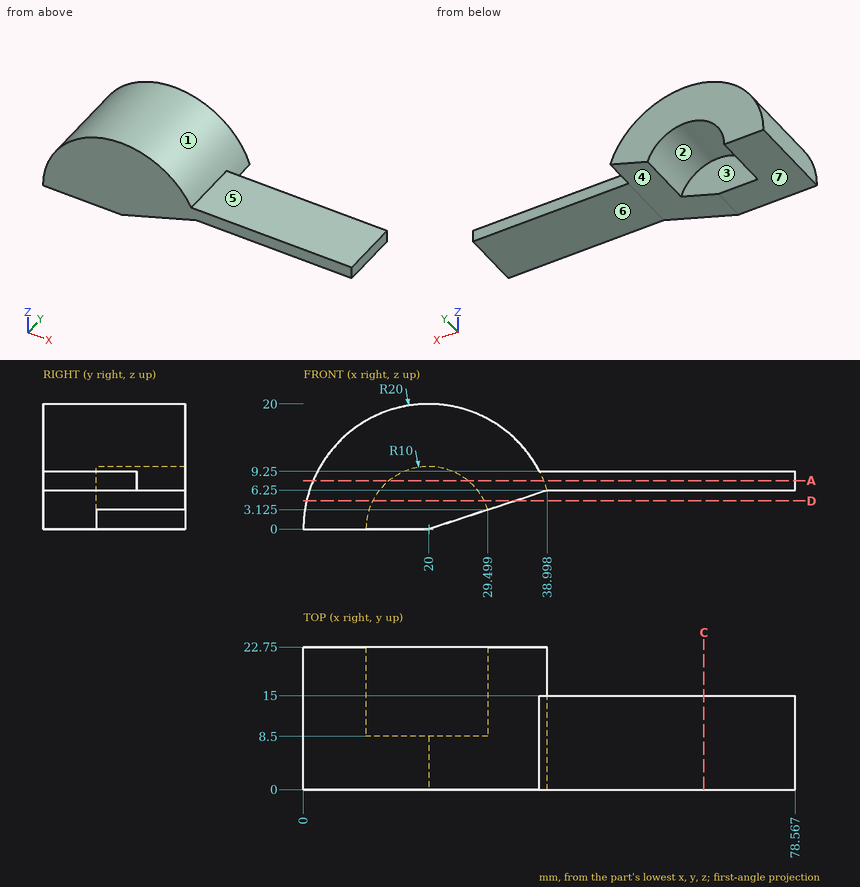
Verification items for this drawing (mm, ordinates from the low corner). A direction names the side the tool comes from. Round coordinates to 2 decimals unless told otherwise and drop trailing zeros. Write each loop counter-clockwise with the first axis right and the second up, starting at its lowest first coordinate (ties: lowest second). Pieces come first, ordered by that corner, then holes. Notation, with made-up numbers: (-2, -0.75) - (16, -0.75) arc R14 ccw to (16, 18.25) - close; hole circle Ø6 at (-25.5, 37). An arc over 180 degrees is marked (long way). One line per item, written item: value.
1. Depth check by flat-ended pin: pin 1 Ø4.5 at (x, y) = (66, 8) entering from -Z; pin 2 Ø1.5 at (x, y) = (30, 2.5) entering from +Z; pin 3 Ø8 at (x, z) = (43, 7) entering from +Y; pin 4 Ø8 at (x, z) = (16, 6.5) entering from +Y. Enter the tip coordinate at first touch or a pass-through.
The answers:
pin 1: stops at z = 6.25
pin 2: stops at z = 17.73
pin 3: stops at y = 15
pin 4: stops at y = 22.75
2. Cross-section at A-A on z = 7.75. Record the boundary of the cut face in (x, y).
The answers:
outline: (1.56, 0) - (78.57, 0) - (78.57, 15) - (38.44, 15) - (38.44, 22.75) - (26.32, 22.75) - (26.32, 8.5) - (13.68, 8.5) - (13.68, 22.75) - (1.56, 22.75) - close
3. Set-up check for the marked faces 5, 6 and 7: record each of +Z, -Z, +X, -X, +Y, -Y from which the full face is reachable in a straight line by a thin tool's end or side.
The answers:
face 5: +Z, +X, +Y, -Y
face 6: -Z, +X, +Y, -Y
face 7: -Z, +X, -X, +Y, -Y
4. Scan lines: L1, parallel to Y at x = 16.5, z = 2.25; L2, parallel to Z at x = 65, y = 13; L3, parallel to Y at x = 48, z = 7.5. Record each from-to range of solid material in increasing order.
The answers:
L1: y = 0 to 8.5
L2: z = 6.25 to 9.25
L3: y = 0 to 15
5. Cross-section at D-D on z = 4.5. Record the boundary of the cut face in (x, y), and give its area (3 significant figures).
The answers:
outline: (0.51, 0) - (33.68, 0) - (33.68, 22.75) - (28.93, 22.75) - (28.93, 8.5) - (11.07, 8.5) - (11.07, 22.75) - (0.51, 22.75) - close
area: 500 mm^2
6. Cross-section at C-C on x = 64. Record the boundary of the cut face in (y, z), and give its area (3 significant figures).
The answers:
outline: (0, 6.25) - (15, 6.25) - (15, 9.25) - (0, 9.25) - close
area: 45.0 mm^2
7. Mould release check, pull along X, two halves, no side actions. Record for the marked faces 1, 2, 3 and 4: released by +X, released by -X, zero draft, split by the parting line, or undercut.
The answers:
face 1: split by the parting line
face 2: undercut
face 3: undercut
face 4: released by +X
